from build123d import *

# Parameters (mm, degrees)
F1_DEPTH = 20
F2_W     = 30
F2_H     = 20
F3_DEPTH = 40


with BuildPart() as f1:
    # F0 (on Top) → F1 (new body)
    with BuildSketch(Plane.XY):
        Polygon((-20, 0), (0, 0), (0, 20), (-60, 20), (-60, 0), (-40, 0), (-40, 10), (-20, 10), align=None)
    extrude(amount=F1_DEPTH)

    # F2 (on face) → F3 (join)
    with BuildSketch(Plane(origin=(0, 0, 0), x_dir=(1, 0, 0), z_dir=(0, 0, -1))):
        with Locations((-45, -30)):
            Rectangle(F2_W, F2_H)
    extrude(amount=-F3_DEPTH)


solid = f1.part
The listing builds one solid part. Answer for the finished solid, in the listing's coordinates (mm). A direction names the side the tool comes from. Coordinates: 2 decimals unless noted, no trailing zeros. Loops run counter-clockwise (first coordinate to the right, second up) from the corner with the lowest first, then second, coordinate; pieces in that order, holes last.
1) Find the intervals of material crossed by L1, parallel to X at y = 8.5, z = 15.5; L2, parallel to X at y = 34, z = 3; L3, parallel to Z at x = -37, y = 16.5, in increasing order.
2) A tool of negligible diameter and unlimited length cuts with its end or side. For faces 4 (the face through (-15, 20, 10)), 5 (the face through (-50, 0, 10)), 6 (the face through (-45, 20, 30)), 7 (the face through (-30, 10, 10)), from which of +Z, -Z, +X, -X, +Y, -Y can it reach the whole face along a straight path? Write none if from no direction.
3) Find section A-A on y = 6. Write down the section's boundary in (x, z).
4) Determine the mould class of faces 1 (the face through (-60, 25, 15)), 2 (the face through (-40, 5, 10)), 3 (the face through (-30, 12, 20)) for opening direction X: pulls with the +X half, pulls with the -X half, needs draft (parallel to the pull), parting line crosses it, or undercut.
5) Find section C-C on x = -32. Write down the section's boundary in (y, z), then the cut area to 3 significant figures.
6) Find section B-B on z = 14.5. Write down the section's boundary in (x, y).
7) Find section D-D on y = 29. Write down the section's boundary in (x, z).
8) Flat-ended cylindrical pins translate along their axes: pin 1 Ø22 at (y, z) = (32, 24.5) entering from +X; pin 2 Ø3 at (x, z) = (-18.5, 10.5) entering from -Y; pin 3 Ø5 at (x, y) = (-19, 8.5) entering from +Z. Find the tip coordinate at first contact, or state that the pin passes through.
Values:
1. L1: x = -60 to -40, -20 to 0
1. L2: x = -60 to -30
1. L3: z = 0 to 20
2. face 4: +Z, -Z, +X, +Y
2. face 5: +Z, -Z, +X, -X, -Y
2. face 6: +Z, +X, -X, -Y
2. face 7: +Z, -Z, -Y
3. outline: (-60, 0) - (-40, 0) - (-40, 20) - (-60, 20) - close; (-20, 0) - (0, 0) - (0, 20) - (-20, 20) - close
4. face 1: pulls with the -X half
4. face 2: undercut
4. face 3: needs draft
5. outline: (10, 0) - (40, 0) - (40, 40) - (20, 40) - (20, 20) - (10, 20) - close
5. area: 1,000 mm2
6. outline: (-60, 0) - (-40, 0) - (-40, 10) - (-20, 10) - (-20, 0) - (0, 0) - (0, 20) - (-30, 20) - (-30, 40) - (-60, 40) - close
7. outline: (-60, 0) - (-30, 0) - (-30, 40) - (-60, 40) - close
8. pin 1: stops at x = -30
8. pin 2: stops at y = 0
8. pin 3: stops at z = 20
